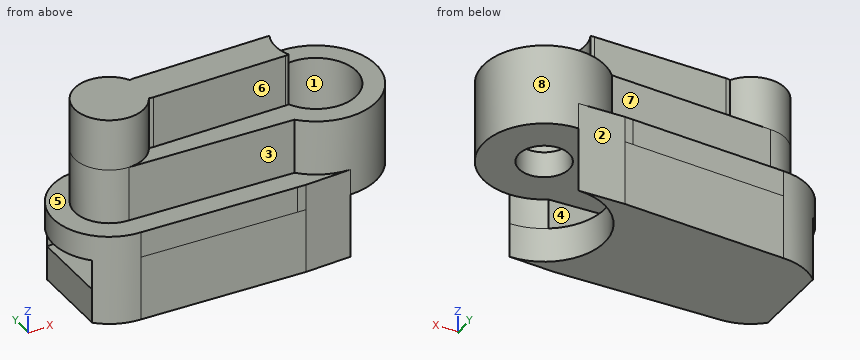
```python
from build123d import *
from build123d.topology import SkipClean

# Parameters (mm, degrees)
SKETCH1_R           = 2.35
BOSS_EXTRUDE1_DEPTH = 6.7
BOSS_EXTRUDE2_DEPTH = 3
CUT_EXTRUDE1_DEPTH  = 2
SKETCH4_R           = 2.35
SKETCH4_R_2         = 1.45
BOSS_EXTRUDE3_DEPTH = 1.5
BOSS_EXTRUDE4_DEPTH = 1.5
BOSS_EXTRUDE5_START = 1.75
BOSS_EXTRUDE5_DEPTH = 1.75
BOSS_EXTRUDE6_START = 2
BOSS_EXTRUDE6_DEPTH = 2


with BuildPart() as part:
    # Sketch1 → Boss-Extrude1 (new body)
    with BuildSketch(Plane.XY):
        with BuildLine():
            Line((-1.533260445, 2.35), (-10.939517975, 2))
            ThreePointArc((-10.939517975, 2), (-12.939517975, 0), (-10.939517975, -2))
            Line((-10.939517975, -2), (-1.533260445, -2.35))
            ThreePointArc((-1.533260445, -2.35), (4.560482025, 0), (-1.533260445, 2.35))
        make_face()
        with Locations((1.060482025, 0)):
            Circle(SKETCH1_R, mode=Mode.SUBTRACT)
    extrude(amount=BOSS_EXTRUDE1_DEPTH)

    # Sketch2 → Boss-Extrude2 (add)
    with SkipClean():  # the faces are left unmerged after this step: merging them gives an invalid solid
        with BuildSketch(Plane.XY.offset(6.7)):
            with BuildLine():
                Line((-8.939517975, 1), (-1.289517975, 1))
                ThreePointArc((-1.289517975, 1), (-1.18252076, 0.99425932), (-1.076752018, 0.977103192))
                ThreePointArc((-1.076752018, 0.977103192), (-1.289517975, 0), (-1.076752018, -0.977103192))
                ThreePointArc((-1.076752018, -0.977103192), (-1.18252076, -0.99425932), (-1.289517975, -1))
                Line((-1.289517975, -1), (-8.939517975, -1))
                ThreePointArc((-8.939517975, -1), (-9.065522268, -0.992029696), (-9.189517975, -0.968245837))
                ThreePointArc((-9.189517975, -0.968245837), (-12.939517975, 0), (-9.189517975, 0.968245837))
                ThreePointArc((-9.189517975, 0.968245837), (-9.065522268, 0.992029696), (-8.939517975, 1))
            make_face()
        extrude(amount=BOSS_EXTRUDE2_DEPTH)

    # Sketch3 → Cut-Extrude1 (cut)
    with SkipClean():  # the faces are left unmerged after this step: merging them gives an invalid solid
        with BuildSketch(Plane(origin=(0, 0, 0), x_dir=(-1, 0, 0), z_dir=(0, 0, -1))):
            with BuildLine():
                Line((10.939517975, 2), (1.533260445, 2.35))
                ThreePointArc((1.533260445, 2.35), (-4.560482025, 0), (1.533260445, -2.35))
                Line((1.533260445, -2.35), (10.939517975, -2))
                ThreePointArc((10.939517975, -2), (12.939517975, 0), (10.939517975, 2))
            make_face()
        extrude(amount=-CUT_EXTRUDE1_DEPTH, mode=Mode.SUBTRACT)

    # Sketch4 → Boss-Extrude3 (add)
    with SkipClean():  # the faces are left unmerged after this step: merging them gives an invalid solid
        with BuildSketch(Plane(origin=(0, 0, 2), x_dir=(-1, 0, 0), z_dir=(0, 0, -1))):
            with Locations((-1.060482025, 0)):
                Circle(SKETCH4_R)
            with Locations((-1.060482025, 0)):
                Circle(SKETCH4_R_2, mode=Mode.SUBTRACT)
        extrude(amount=-BOSS_EXTRUDE3_DEPTH)

    # Sketch5 → Boss-Extrude4 (add)
    with SkipClean():  # the faces are left unmerged after this step: merging them gives an invalid solid
        with BuildSketch(Plane(origin=(0, 0, 2), x_dir=(-1, 0, 0), z_dir=(0, 0, -1))):
            with BuildLine():
                Line((-1.060482025, -3.5), (1.579739871, -3.599135566))
                Line((1.579739871, -3.599135566), (2.059938037, -3.581267742))
                Line((2.059938037, -3.581267742), (10.965572511, -3.249895562))
                ThreePointArc((10.965572511, -3.249895562), (14.189517975, 0), (10.965572511, 3.249895562))
                Line((10.965572511, 3.249895562), (2.059938037, 3.581267742))
                Line((2.059938037, 3.581267742), (1.579739871, 3.599135566))
                Line((1.579739871, 3.599135566), (-1.060482025, 3.5))
                ThreePointArc((-1.060482025, 3.5), (0.358144071, 3.199609351), (1.533260445, 2.35))
                Line((1.533260445, 2.35), (10.939517975, 2))
                ThreePointArc((10.939517975, 2), (12.939517975, 0), (10.939517975, -2))
                Line((10.939517975, -2), (1.533260445, -2.35))
                ThreePointArc((1.533260445, -2.35), (0.358144071, -3.199609351), (-1.060482025, -3.5))
            make_face()
        extrude(amount=-BOSS_EXTRUDE4_DEPTH)

    # Sketch7 → Boss-Extrude5 (add)
    with SkipClean():  # the faces are left unmerged after this step: merging them gives an invalid solid
        with BuildSketch(Plane(origin=(0, 0, 2), x_dir=(-1, 0, 0), z_dir=(0, 0, -1)).offset(BOSS_EXTRUDE5_START)):
            with BuildLine():
                ThreePointArc((10.965572511, -3.249895562), (12.19945489, -2.995840278), (13.244032441, -2.291661642))
                Line((13.244032441, -2.291661642), (0.86770197, -2.920976974))
                ThreePointArc((0.86770197, -2.920976974), (-0.05385881, -3.35212018), (-1.060482025, -3.5))
                Line((-1.060482025, -3.5), (1.579739871, -3.599135566))
                Line((1.579739871, -3.599135566), (10.965572511, -3.249895562))
            make_face()
            with BuildLine():
                Line((0.86770197, 2.920976974), (13.244032441, 2.291661642))
                ThreePointArc((13.244032441, 2.291661642), (12.19945489, 2.995840278), (10.965572511, 3.249895562))
                Line((10.965572511, 3.249895562), (1.579739871, 3.599135566))
                Line((1.579739871, 3.599135566), (-1.060482025, 3.5))
                ThreePointArc((-1.060482025, 3.5), (-0.05385881, 3.35212018), (0.86770197, 2.920976974))
            make_face()
        extrude(amount=-BOSS_EXTRUDE5_DEPTH)

    # Sketch8 → Boss-Extrude6 (add)
    with SkipClean():  # the faces are left unmerged after this step: merging them gives an invalid solid
        with BuildSketch(Plane(origin=(0, 0, 0.25), x_dir=(-1, 0, 0), z_dir=(0, 0, -1)).offset(BOSS_EXTRUDE6_START)):
            with BuildLine():
                Line((10.965572511, 3.249895562), (1.579739871, 3.599135566))
                Line((1.579739871, 3.599135566), (-1.060482025, 3.5))
                ThreePointArc((-1.060482025, 3.5), (2.439517975, 0), (-1.060482025, -3.5))
                Line((-1.060482025, -3.5), (1.579739871, -3.599135566))
                Line((1.579739871, -3.599135566), (10.965572511, -3.249895562))
                ThreePointArc((10.965572511, -3.249895562), (12.19945489, -2.995840278), (13.244032441, -2.291661642))
                Line((13.244032441, -2.291661642), (13.244032441, 2.291661642))
                ThreePointArc((13.244032441, 2.291661642), (12.19945489, 2.995840278), (10.965572511, 3.249895562))
            make_face()
        extrude(amount=-BOSS_EXTRUDE6_DEPTH)


solid = part.part
```
The listing builds one solid part. Answer for the finished solid, in the listing's coordinates (mm). Face numbers are marked on the shaded views. A direction names the side the tool comes from. Round coordinates to 2 decimals unless told otherwise and drop trailing zeros. Order: outer loops, then holes, each group sorted by start corner. A loop starts at its lowest first (then second) coordinate and runs counter-clockwise, first axis right, second up. Notation, with made-up numbers: (-39.5, 35) -> (5.5, 35) arc R24 cw to (5.5, 53) -> close; hole circle Ø3 at (-35.75, -3). An arc over 180 degrees is marked (long way). Answer as CSV lines item,"result".
Q1. A cutting plane is placed at A-A on z = 2.5. Determine the outline of the cut face in (x, y).
Computed values:
outline,"(-10.97, -3.25) -> (-1.58, -3.6) -> (1.06, -3.5) arc R3.5 ccw to (1.06, 3.5) -> (-1.58, 3.6) -> (-10.97, 3.25) arc R3.25 ccw to start; hole circle Ø2.9 at (1.06, 0)"
Q2. Which of the six approach directions +Z, -Z, +X, -X, +Y, -Y give full straight-line access (tool end or side, diameter ignored) to the marked faces 4, 5, 6, 7 and 8?
Computed values:
face 4,"+X"
face 5,"+Z, -X"
face 6,"+Z, +X, -Y"
face 7,"+Z, -X, +Y"
face 8,"+Z"
Q3. A cutting plane is placed at C-C on x = -3. Determine the outline of the cut face in (y, z), plus the area to 3 significant figures.
Computed values:
outline,"(-3.55, -1.75) -> (3.55, -1.75) -> (3.55, 3.5) -> (2.3, 3.5) -> (2.3, 6.7) -> (1, 6.7) -> (1, 9.7) -> (-1, 9.7) -> (-1, 6.7) -> (-2.3, 6.7) -> (-2.3, 3.5) -> (-3.55, 3.5) -> close; hole (-2.81, 0.25) -> (2.81, 0.25) -> (2.81, 2) -> (-2.81, 2) -> close"
area,"48.1 mm^2"
Q4. A cutting plane is placed at B-B on y = 0. Determine the outline of the cut face in (x, z), plus the area to 3 significant figures.
Computed values:
outline,"(-14.19, 2) -> (-0.39, 2) -> (-0.39, 3.5) -> (-1.29, 3.5) -> (-1.29, 9.7) -> (-12.94, 9.7) -> (-12.94, 3.5) -> (-14.19, 3.5) -> close; (-13.24, -1.75) -> (-2.44, -1.75) -> (-2.44, 0.25) -> (-13.24, 0.25) -> close; (2.51, 2) -> (4.56, 2) -> (4.56, 6.7) -> (3.41, 6.7) -> (3.41, 3.5) -> (2.51, 3.5) -> close"
area,"121 mm^2"
Q5. A cutting plane is placed at D-D on z = 0. Determine the outline of the cut face in (x, y).
Computed values:
outline,"(-13.24, -2.29) arc R3.25 ccw to (-10.97, -3.25) -> (-1.58, -3.6) -> (1.06, -3.5) arc R3.5 cw to (1.06, 3.5) -> (-1.58, 3.6) -> (-10.97, 3.25) arc R3.25 ccw to (-13.24, 2.29) -> close"
Q6. Given pin 1 (2.5 mm diameter, centred on x = -5.5, z = 8.5, fed in from -Y); pin 2 (3.5 mm diameter, centred on x = -1, y = -1.5, fed in from +Z); pin 3 (3.5 mm diameter, centred on x = 1.06, y = 0, fed in from -Z); pin 4 (0.9 mm diameter, centred on x = -6.5, z = 8.5, fed in from +Y), each flat-ended and moving along its own axis, determine where each tip first touches the part or whether it passes through.
Computed values:
pin 1,"stops at y = -1"
pin 2,"stops at z = 9.7"
pin 3,"stops at z = 2"
pin 4,"stops at y = 1"
Q7. For a pull along X with two mould halves and no side action, classify the marked faces 1, 2 and 3 as +X half, -X half, draft (parallel to the pull), parting line (faces both ways), or undercut.
Computed values:
face 1,"undercut"
face 2,"+X half"
face 3,"-X half"
Q8. Consider line 1 (Z direction, x = -3, y = -1.25); line 2 (Z direction, x = -6.5, y = 0.5); line 3 (X direction, y = 0, z = 6.5). Determine where each line is inside the solid, lowest interval first. Write a range as from..to.
Computed values:
line 1,"z = -1.75..0.25, 2..6.7"
line 2,"z = -1.75..0.25, 2..9.7"
line 3,"x = -12.94..-1.29, 3.41..4.56"
